Can you work these out from the model? Positions are in its coordinate system, mm. A direction names the side the tool comes from. Give positions to 0.01 mm unless a question says otherwise; leave off trailing zeros. Order: outer loops, then holes, each group sorted by start corner. A loop starts at its lowest first (then second) coordinate and runs counter-clockwise, first axis right, second up. Notation, with made-up numbers: M 56,80 L 80,80 A23 cw 80,100 Z; hole C 35.25,-31.5 d7. An arc over 180 degrees is marked long. Write each question's results on one line, items separated by ' | '.
from build123d import *

# Parameters (mm, degrees)
SKETCH2_W           = 38
SKETCH2_H           = 170
SKETCH2_R           = 1.5
SKETCH2_W_2         = 2
SKETCH2_H_2         = 6
SKETCH2_W_3         = 55
SKETCH2_H_3         = 58.475280412
BOSS_EXTRUDE2_DEPTH = 3
BOSS_EXTRUDE3_DEPTH = 10
SKETCH2_4_R         = 15
BOSS_EXTRUDE4_DEPTH = 25
SKETCH3_R           = 65
BOSS_EXTRUDE5_DEPTH = 7
SKETCH4_W           = 26
SKETCH4_H           = 54
SKETCH4_H_2         = 15.857774488
BOSS_EXTRUDE6_DEPTH = 30
SKETCH5_W           = 38
SKETCH5_H           = 158.814442682
BOSS_EXTRUDE7_DEPTH = 4
DRAFT1_ANGLE        = -20
SKETCH6_R           = 0.5
CUT_EXTRUDE1_DEPTH  = 1


with BuildPart() as part:
    # Sketch2 → Boss-Extrude2 (new body)
    with BuildSketch(Plane(origin=(0, 0, 0), x_dir=(1, 0, 0), z_dir=(0, 1, 0))):
        with Locations((0, 8)):
            Rectangle(SKETCH2_W, SKETCH2_H)
        with Locations((-13, -72)):
            Circle(SKETCH2_R, mode=Mode.SUBTRACT)
        with Locations((13, -72)):
            Circle(SKETCH2_R, mode=Mode.SUBTRACT)
        with Locations((13, -40)):
            Rectangle(SKETCH2_W_2, SKETCH2_H_2, mode=Mode.SUBTRACT)
        with Locations((-13.416960254, -40)):
            Rectangle(SKETCH2_W_2, SKETCH2_H_2, mode=Mode.SUBTRACT)
        Rectangle(SKETCH2_W_3, SKETCH2_H_3)
        with Locations((-25.5, 20)):
            Circle(SKETCH2_R, mode=Mode.SUBTRACT)
        with Locations((25.5, 20)):
            Circle(SKETCH2_R, mode=Mode.SUBTRACT)
        with Locations((25.5, -20)):
            Circle(SKETCH2_R, mode=Mode.SUBTRACT)
        with Locations((-25.5, -20)):
            Circle(SKETCH2_R, mode=Mode.SUBTRACT)
    extrude(amount=BOSS_EXTRUDE2_DEPTH)

    # Sketch2<3> → Boss-Extrude3 (add)
    with BuildSketch(Plane(origin=(0, 0, 0), x_dir=(1, 0, 0), z_dir=(0, 1, 0))):
        with BuildLine():
            ThreePointArc((-90.482980764, 78.72426795), (-93.205224918, 73.232676721), (-97.896839388, 69.288447884))
            Line((-97.896839388, 69.288447884), (-27.5, 13.976645508))
            Line((-27.5, 13.976645508), (-27.5, 29.237640206))
            Line((-27.5, 29.237640206), (-90.482980764, 78.72426795))
        make_face()
        with BuildLine():
            Line((-27.5, -13.976645508), (-97.896839388, -69.288447884))
            ThreePointArc((-97.896839388, -69.288447884), (-93.205224918, -73.232676721), (-90.482980764, -78.72426795))
            Line((-90.482980764, -78.72426795), (-27.5, -29.237640206))
            Line((-27.5, -29.237640206), (-27.5, -13.976645508))
        make_face()
        with BuildLine():
            Line((90.482980764, 78.72426795), (27.5, 29.237640206))
            Line((27.5, 29.237640206), (27.5, 13.976645508))
            Line((27.5, 13.976645508), (97.896839388, 69.288447884))
            ThreePointArc((97.896839388, 69.288447884), (93.205224918, 73.232676721), (90.482980764, 78.72426795))
        make_face()
        with BuildLine():
            Line((27.5, -29.237640206), (90.482980764, -78.72426795))
            ThreePointArc((90.482980764, -78.72426795), (93.205224918, -73.232676721), (97.896839388, -69.288447884))
            Line((97.896839388, -69.288447884), (27.5, -13.976645508))
            Line((27.5, -13.976645508), (27.5, -29.237640206))
        make_face()
    extrude(amount=BOSS_EXTRUDE3_DEPTH)

    # Sketch2<4> → Boss-Extrude4 (add)
    with BuildSketch(Plane(origin=(0, 0, 0), x_dir=(1, 0, 0), z_dir=(0, 1, 0))):
        with Locations((-105, 82.5)):
            Circle(SKETCH2_4_R)
        with Locations((105, 82.5)):
            Circle(SKETCH2_4_R)
        with Locations((105, -82.5)):
            Circle(SKETCH2_4_R)
        with Locations((-105, -82.5)):
            Circle(SKETCH2_4_R)
    extrude(amount=BOSS_EXTRUDE4_DEPTH)

    # Sketch3 → Boss-Extrude5 (add)
    with BuildSketch(Plane(origin=(0, 25, 0), x_dir=(1, 0, 0), z_dir=(0, 1, 0))):
        with Locations((-105, -82.5)):
            Circle(SKETCH3_R)
        with Locations((105, -82.5)):
            Circle(SKETCH3_R)
        with Locations((105, 82.5)):
            Circle(SKETCH3_R)
        with Locations((-105, 82.5)):
            Circle(SKETCH3_R)
    extrude(amount=BOSS_EXTRUDE5_DEPTH)

    # Sketch4 → Boss-Extrude6 (add)
    with BuildSketch(Plane(origin=(0, 3, 0), x_dir=(1, 0, 0), z_dir=(0, 1, 0))):
        Rectangle(SKETCH4_W, SKETCH4_H)
        with Locations((0, 78.679384084)):
            Rectangle(SKETCH4_W, SKETCH4_H_2)
    extrude(amount=BOSS_EXTRUDE6_DEPTH)

    # Sketch5 → Boss-Extrude7 (add)
    with BuildSketch(Plane(origin=(0, 33, 0), x_dir=(1, 0, 0), z_dir=(0, 1, 0))):
        with Locations((0, 2.407221341)):
            Rectangle(SKETCH5_W, SKETCH5_H)
    extrude(amount=BOSS_EXTRUDE7_DEPTH)

    # Draft1
    draft1_faces = [part.faces().sort_by_distance(p)[0] for p in [
        (0, 18, -86.608271328),
    ]]
    draft(draft1_faces, Plane.ZX.offset(33), DRAFT1_ANGLE)

    # Sketch6 → Cut-Extrude1 (cut)
    with BuildSketch(Plane.XZ):
        Circle(SKETCH6_R)
    extrude(amount=-CUT_EXTRUDE1_DEPTH, mode=Mode.SUBTRACT)


solid = part.part
(1) Imagine slicing it at C-C, the plane x = -75.5. Write out the boundary of the cut face in (y, z).
Data:
outline: M 0,-66.95 L 10,-66.95 L 10,-51.69 L 0,-51.69 Z; M 0,51.69 L 10,51.69 L 10,66.95 L 0,66.95 Z; M 25,-140.42 L 32,-140.42 L 32,-24.58 L 25,-24.58 Z; M 25,24.58 L 32,24.58 L 32,140.42 L 25,140.42 Z
(2) Imagine slicing it at D-D, the plane z = -37.5. Write out the boundary of the cut face in (x, y).
Data:
outline: M -151.9,25 L -58.1,25 L -58.1,32 L -151.9,32 Z; M -57.44,0 L -38.02,0 L -38.02,10 L -57.44,10 Z; M -19,0 L 19,0 L 19,3 L -19,3 Z; M -19,33 L 19,33 L 19,37 L -19,37 Z; M 38.02,0 L 57.44,0 L 57.44,10 L 38.02,10 Z; M 58.1,25 L 151.9,25 L 151.9,32 L 58.1,32 Z
(3) Imagine slicing it at A-A, the plane x = 105. Write out the boundary of the cut face in (y, z), plus the area to 3 significant figures.
Data:
outline: M 0,-97.5 L 25,-97.5 L 25,-147.5 L 32,-147.5 L 32,-17.5 L 25,-17.5 L 25,-67.5 L 0,-67.5 Z; M 0,67.5 L 25,67.5 L 25,17.5 L 32,17.5 L 32,147.5 L 25,147.5 L 25,97.5 L 0,97.5 Z | area: 3,320 mm2
(4) Imagine slicing it at B-B, the plane z = 120. Write out the boundary of the cut face in (x, y).
Data:
outline: M -158.09,25 L -51.91,25 L -51.91,32 L -158.09,32 Z; M 51.91,25 L 158.09,25 L 158.09,32 L 51.91,32 Z
(5) We'd pull the mould along X, two halves only. Please class faces 1 (the face through (-106, 32, -83)), 2 (the face through (-116.9, 12.32, 91.63)): +X half, -X half, draft (parallel to the pull), parting line (faces both ways), or undercut.
Data:
face 1: draft | face 2: undercut
(6) Will these pins go through, and if not, where does the flat tip stop? P1, Ø1.5, axis at x = -77.5, z = -91.5, coming from the -Y side; P2, Ø13, axis at x = -3.5, y = 17, coming from the +Z side; P3, Ø1.5, axis at x = -23, y = 1.5, coming from the -Z side; P4, Ø1.5, axis at x = -18, z = 72.5, coming from the -Y side.
Data:
P1: stops at y = 25 | P2: stops at z = 27 | P3: stops at z = -29.24 | P4: stops at y = 0
(7) For faces 3 (the face through (0, 18, -27)), 4 (the face through (-0.182, 17.79, -81.072)), 5 (the face through (13, 18, 0)), which set-ups out of +Z, -Z, +X, -X, +Y, -Y let a thin tool reach every point of the face, with its end or its side?
Data:
face 3: none | face 4: -Z | face 5: +Z, -Z
(8) I need wall thicknesses on L1, parallel to Z at x = -25.5, y = 1; L2, parallel to Z at x = 13, y = 2.1; L3, parallel to X at y = 2, z = 20. Which ranges of each line are inside material? Lowest first, please. Write a range as from..to.
Data:
L1: z = -29.24..-21.5, -18.5..18.5, 21.5..29.24 | L2: z = -93..37, 43..70.5, 73.5..77 | L3: x = -35.17..-27, -24..24, 27..35.17
